Could you check a few things on this drawing? It's one solid part, dimensions in mm from its lowest x, y, z. Round coordinates to 2 decimals unless told otherwise and drop trailing zeros. Order: outer loops, then holes, each group sorted by start corner. A loop starts at its lowest first (then second) coordinate and runs counter-clockwise, first axis right, second up. Notation, with made-up numbers: (26, -23.75) -> (32, -23.75) arc R30 cw to (32, 0.25) -> close; hole circle Ø6 at (8, -26.5). An arc over 180 degrees is marked (long way). Use a Markdown table: item, result. Add a question column.
(1) I want a section at C-C, the plane y = 11. Please give me the cut outline in (x, z), then the cut area to 3 significant figures.
(2) I want a section at B-B, the plane x = 38.1. Please give me the cut outline in (y, z).
(3) Thinking about a two-plate mould opening in X: for the marked faces 1, 2, 3 and 4, which applies, pulls with the +X half, pulls with the -X half, needs draft (parallel to the pull), parting line crosses it, or undercut?
(4) I want a section at A-A, the plane z = 38.1. Please give me the cut outline in (x, y).
(5) I'm going to push a flat-ended pin straight in: P1, Ø6, axis at y = 28.5, z = 68.5, coming from the -X side. Where does the tip first touch, or does it pass through?
(6) If I drill on probe 1 along X at (y, z) = (12, 38); probe 2 along Z at (x, y) = (33, 23), over which ranges is the centre line in solid material (lowest first)?
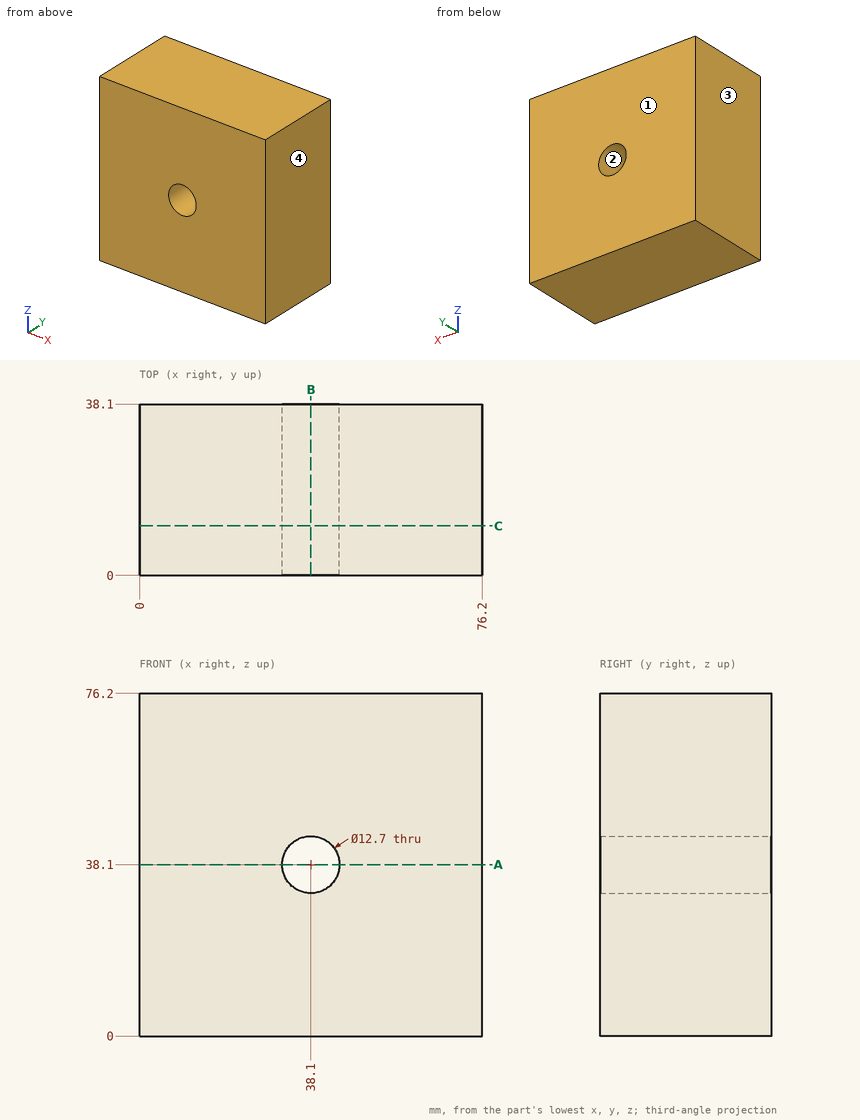
Taken from the geometry:
| question | item | result |
|---|---|---|
| 1 | outline | (0, 0) -> (76.2, 0) -> (76.2, 76.2) -> (0, 76.2) -> close; hole circle Ø12.7 at (38.1, 38.1) |
| 1 | area | 5,680 mm2 |
| 2 | outline | (0, 0) -> (38.1, 0) -> (38.1, 31.75) -> (0, 31.75) -> close; (0, 44.45) -> (38.1, 44.45) -> (38.1, 76.2) -> (0, 76.2) -> close |
| 3 | face 1 | needs draft |
| 3 | face 2 | undercut |
| 3 | face 3 | pulls with the -X half |
| 3 | face 4 | pulls with the +X half |
| 4 | outline | (0, 0) -> (31.75, 0) -> (31.75, 38.1) -> (0, 38.1) -> close; (44.45, 0) -> (76.2, 0) -> (76.2, 38.1) -> (44.45, 38.1) -> close |
| 5 | P1 | stops at x = 0 |
| 6 | probe 1 | x = 0 to 31.75, 44.45 to 76.2 |
| 6 | probe 2 | z = 0 to 34.32, 41.88 to 76.2 |
